```python
from build123d import *

# Parameters (mm, degrees)
F0_W      = 30
F0_H      = 25
F1_DEPTH  = 2
F2_R      = 1
F3_DEPTH  = 2
F4_W      = 30
F4_H      = 15
F5_DEPTH  = 15
F7_DEPTH  = 15
F9_DEPTH  = 15
F10_R     = 5.15
F11_DEPTH = 28.2428712579
F12_R     = 1


with BuildPart() as f1:
    # F0 (on Top) → F1 (new body)
    with BuildSketch(Plane.XY):
        Rectangle(F0_W, F0_H)
    extrude(amount=F1_DEPTH)

    # F2 (on face) → F3 (cut)
    with BuildSketch(Plane.XY.offset(2)):
        with Locations((12.5, 10)):
            Circle(F2_R)
        with Locations((-12.5, 10)):
            Circle(F2_R)
        with Locations((-12.5, -10)):
            Circle(F2_R)
        with Locations((12.5, -10)):
            Circle(F2_R)
    extrude(amount=-F3_DEPTH, mode=Mode.SUBTRACT)

    # F4 (on face) → F5 (join)
    with BuildSketch(Plane.XY.offset(2)):
        Rectangle(F4_W, F4_H)
    extrude(amount=F5_DEPTH)

    # F6 (on face) → F7 (cut, through all)
    with BuildSketch(Plane.XZ.offset(7.5)):
        Polygon((-15, 9.5), (15, 17), (-15, 17), align=None)
    extrude(amount=-F7_DEPTH, mode=Mode.SUBTRACT)

    # F8 (on face) → F9 (cut, through all)
    with BuildSketch(Plane.XZ.offset(7.5)):
        Polygon((15, 2), (15, 17), (12.3550952894, 2), align=None)
    extrude(amount=-F9_DEPTH, mode=Mode.SUBTRACT)

    # F10 (on face) → F11 (cut, through all)
    with BuildSketch(Plane(origin=(11.6405234376, 0, -2.0525383516), x_dir=(0, 1, 0), z_dir=(0.984807753, 0, -0.1736481777))):
        with Locations((0, 10.1150552879)):
            Circle(F10_R)
    extrude(amount=-F11_DEPTH, mode=Mode.SUBTRACT)

    # F12
    f12_edges = [f1.edges().sort_by_distance(p)[0] for p in [
        (13.677548, -7.5, 9.5),
        (13.677548, 7.5, 9.5),
        (15, 0, 17),
    ]]
    fillet(f12_edges, radius=F12_R)


solid = f1.part
```
Model file for the job. Use its own axes, mm. A direction names the side the tool comes from. Give positions to 0.01 mm unless a question says otherwise; leave off trailing zeros. Order: outer loops, then holes, each group sorted by start corner. A loop starts at its lowest first (then second) coordinate and runs counter-clockwise, first axis right, second up.
1) Pin check, flat tips, straight feed: pin 1 (1.8 mm diameter, centred on x = -12.5, y = -10, fed in from +Z); pin 2 (1.5 mm diameter, centred on x = 5, y = 3.5, fed in from +Z); pin 3 (7.5 mm diameter, centred on x = -6.5, z = 7, fed in from +Y); pin 4 (3 mm diameter, centred on y = 0, z = 4, fed in from +X). Stop position of each tip, or through.
2) Saw through at A-A, the plane y = 10. Write the cut outline in (x, z), then the cut area to 3 significant figures.
3) 3-axis set-ups, long thin cutter, end or side, ignore diameter. For faces 1 (the flat face through (-1, 7.5, 8)), 2 (the flat face through (14.353, -0.091, 13.33)), 3 (the flat face through (0, 9, 2)): which of +Z, -Z, +X, -X, +Y, -Y reach the whole face in a straight line?
4) Saw through at B-B, the plane y = -1.5. Write the cut outline in (x, z), then the cut area to 3 significant figures.
5) Saw through at D-D, the plane x = -12.5. Count the separate pieces of the cut face and the enclosed holes in it, then the cut area to 3 significant figures.
6) Wall check: probe 1 along Y at (x, z) = (12.5, 1); probe 2 along Y at (x, z) = (11.5, 3.75); probe 3 along Y at (x, z) = (8, 10.5). Give the ranges that are in metal, low to high.
7) Mould opens along X. For faces 4 (the flat face through (5.4, -1.8, 14.6)), 5 (the cylindrical face through (13.301, 7.215, 9.097)), 6 (the cylindrical face through (12.37, -9.01, 1.01)), 7 (the flat face through (-1, -7.5, 8)) say: +X half, -X half, draft (parallel to the pull), parting line (faces both ways), or undercut.
8) Saw through at C-C, the plane y = 7. Write the cut outline in (x, z).
Computed:
1. pin 1: passes through
1. pin 2: stops at z = 14.69
1. pin 3: stops at y = 7.5
1. pin 4: stops at x = 12.52
2. outline: (-15, 0) - (-13.5, 0) - (-13.5, 2) - (-15, 2) - close; (-11.5, 0) - (11.5, 0) - (11.5, 2) - (-11.5, 2) - close; (13.5, 0) - (15, 0) - (15, 2) - (13.5, 2) - close
2. area: 52.0 mm2
3. face 1: +Z, +X, -X, +Y
3. face 2: +X, +Y, -Y
3. face 3: +X
4. outline: (-15, 0) - (15, 0) - (15, 2) - (12.36, 2) - (12.54, 3.06) - (-15, 7.91) - close; (4.75, 14.44) - (14.25, 12.76) - (14.73, 15.48) arc R1 ccw to (13.51, 16.63) - close
4. area: 176 mm2
5. separate pieces: 3
5. enclosed holes: 0
5. area: 145 mm2
6. probe 1: y = -12.5 to -11, -9 to 9, 11 to 12.5
6. probe 2: y = -7.5 to -2.63, 2.63 to 7.5
6. probe 3: y = -7.5 to -4.89, 4.89 to 7.5
7. face 4: -X half
7. face 5: +X half
7. face 6: undercut
7. face 7: draft
8. outline: (-15, 0) - (15, 0) - (15, 2) - (12.22, 2) - (14.69, 16) arc R1 ccw to (13.51, 16.63) - (-15, 9.5) - close
